Design review of the part built by this model. Coordinates are the model's own, in mm. A direction names the side the tool comes from. Coordinates: 2 decimals unless noted, no trailing zeros. Loops run counter-clockwise (first coordinate to the right, second up) from the corner with the lowest first, then second, coordinate; pieces in that order, holes last. Notation, with made-up numbers: (15.5, -8) -> (63.5, -8) arc R31 ccw to (63.5, 19) -> close; hole circle Ø6 at (70, 75.25). An arc over 180 degrees is marked (long way). Answer as a JSON object with one key per item and string values.
```python
from build123d import *

# Parameters (mm, degrees)
ESQUISSE2_R                  = 20.5
EXTRUSION1_DEPTH             = 4.8
ESQUISSE3_R                  = 6.25
EXTRUSION2_DEPTH             = 10
ENL_V_MAT_EXTRU_1_DEPTH      = 10
ESQUISSE5_R                  = 1.5
ENL_V_MAT_EXTRU_2_DEPTH      = 33.550576032
ESQUISSE6_R                  = 6.4
ENL_V_MAT_EXTRU_3_DEPTH      = 1.8
ESQUISSE7_R                  = 1
ENL_V_MAT_EXTRU_4_DEPTH      = 1
ENL_V_MAT_EXTRU_5_DEPTH      = 1.8
R_P_TITION_CIRCULAIRE1_COUNT = 6


with BuildPart() as part:
    # Esquisse2 → Extrusion1 (new body)
    with BuildSketch(Plane.XY):
        Circle(ESQUISSE2_R)
    extrude(amount=EXTRUSION1_DEPTH)

    # Esquisse3 → Extrusion2 (add)
    with BuildSketch(Plane.XY.offset(4.8)):
        with Locations((-3.25, 0)):
            Circle(ESQUISSE3_R)
    extrude(amount=EXTRUSION2_DEPTH)

    # Esquisse4 → Enl_v. mat.-Extru.1 (cut)
    with BuildSketch(Plane.XY.offset(14.8)):
        with BuildLine():
            ThreePointArc((0.388846154, 2.974693038), (-3, 0), (0.388846154, -2.974693038))
            ThreePointArc((0.388846154, -2.974693038), (-7.95, 0), (0.388846154, 2.974693038))
        make_face()
    extrude(amount=-ENL_V_MAT_EXTRU_1_DEPTH, mode=Mode.SUBTRACT)

    # Esquisse5 → Enl_v. mat.-Extru.2 (cut, through all)
    with BuildSketch(Plane.XY.offset(14.8)):
        Circle(ESQUISSE5_R)
    extrude(amount=-ENL_V_MAT_EXTRU_2_DEPTH, mode=Mode.SUBTRACT)

    # Esquisse6 → Enl_v. mat.-Extru.3 (cut)
    with BuildSketch(Plane(origin=(0, 0, 0), x_dir=(-1, 0, 0), z_dir=(0, 0, -1))):
        Circle(ESQUISSE6_R)
    extrude(amount=-ENL_V_MAT_EXTRU_3_DEPTH, mode=Mode.SUBTRACT)

    # Esquisse7 → Enl_v. mat.-Extru.4 (cut)
    with BuildSketch(Plane.XY.offset(4.8)):
        with Locations((0, 15)):
            Circle(ESQUISSE7_R)
    extrude(amount=-ENL_V_MAT_EXTRU_4_DEPTH, mode=Mode.SUBTRACT)

    # Esquisse8 → Enl_v. mat.-Extru.5 (cut)
    with BuildSketch(Plane(origin=(0, 0, 0), x_dir=(-1, 0, 0), z_dir=(0, 0, -1))):
        with BuildLine():
            Line((-3.190947925, 7.22688393), (-7.708190102, 15.05097689))
            ThreePointArc((-7.708190102, 15.05097689), (0, 16.91), (7.708190102, 15.05097689))
            Line((7.708190102, 15.05097689), (3.190947925, 7.22688393))
            ThreePointArc((3.190947925, 7.22688393), (0, 7.9), (-3.190947925, 7.22688393))
        make_face()
    enl_v_mat_extru_5 = extrude(amount=-ENL_V_MAT_EXTRU_5_DEPTH, mode=Mode.SUBTRACT)

    # R_p_tition circulaire1: Enl_v. mat.-Extru.5 ×6 about axis
    r_p_tition_circulaire1_axis = Axis((0, 0, 0), (0, 0, 1))
    for i in range(1, R_P_TITION_CIRCULAIRE1_COUNT):
        add(enl_v_mat_extru_5.rotate(r_p_tition_circulaire1_axis, i * 360 / R_P_TITION_CIRCULAIRE1_COUNT), mode=Mode.SUBTRACT)


solid = part.part
```
1) Add section C-C, the plane y = -18. Give the boundary of the cut face in (x, z), and give its area (3 significant figures).
Completed:
{"outline": "(-9.81, 0) -> (9.81, 0) -> (9.81, 4.8) -> (-9.81, 4.8) -> close", "area": "94.2 mm²"}
2) Add section B-B, the plane z = 10.25. Give the boundary of the cut face in (x, y).
Completed:
{"outline": "circle Ø12.5 at (-3.25, 0); hole circle Ø3 at (0, 0); hole (0.39, -2.97) arc R3 cw (long way) to (0.39, 2.97) arc R4.7 ccw (long way) to start"}
3) Add section A-A, the plane y = 0. Give the boundary of the cut face in (x, z), and give its area (3 significant figures).
Completed:
{"outline": "(-20.5, 0) -> (-6.4, 0) -> (-6.4, 1.8) -> (-1.5, 1.8) -> (-1.5, 14.8) -> (-3, 14.8) -> (-3, 4.8) -> (-7.95, 4.8) -> (-7.95, 14.8) -> (-9.5, 14.8) -> (-9.5, 4.8) -> (-20.5, 4.8) -> close; (1.5, 1.8) -> (6.4, 1.8) -> (6.4, 0) -> (20.5, 0) -> (20.5, 4.8) -> (3, 4.8) -> (3, 14.8) -> (1.5, 14.8) -> close", "area": "210 mm²"}
4) Clearance check with flat-ended pins moving along their axes: pin 1 Ø3 at (y, z) = (0, 9.5) entering from +X; pin 2 Ø0.5 at (x, z) = (13.5, 1.5) entering from +Y; pin 3 Ø3 at (x, y) = (0, 15) entering from -Z. State where each tip first meets the part, or that it passes through.
Completed:
{"pin 1": "x = 3", "pin 2": "y = 15.64", "pin 3": "z = 1.8"}
5) Wall thickness on probe 1 along Y at (x, z) = (0, 4.6); probe 2 along Y at (x, z) = (-2.5, 8); probe 3 along Y at (x, z) = (-0.5, 5.5): over which ranges is each line inside the solid? List them lowest first.
Completed:
{"probe 1": "-20.5 to -1.5, 1.5 to 14, 16 to 20.5", "probe 2": "-6.2 to -4.64, -1.66 to 1.66, 4.64 to 6.2", "probe 3": "-5.61 to -3.81, -2.96 to -1.41, 1.41 to 2.96, 3.81 to 5.61"}
6) For faces 1 (the flat face through (-2, 0, 14.8)), 2 (the cylindrical face through (14.7, 8.36, 0.89)), list the 3-axis set-ups (+Z, -Z, +X, -X, +Y, -Y) from which the entire face can be reached by the end or side of a thin tool; tool diameter is ignored.
Completed:
{"face 1": "+Z, +X, -X, +Y, -Y", "face 2": "-Z"}
7) The part is to be moulded in two halves that separate along Y. For faces 3 (the flat face through (-10, -6, 1.8)), 4 (the flat face through (4, 0, 4.8)), 5 (the cylindrical face through (-4.444, -20.013, 2.366)), say which applies: pulls with the +Y half, pulls with the -Y half, needs draft (parallel to the pull), parting line crosses it, or undercut.
Completed:
{"face 3": "undercut", "face 4": "needs draft", "face 5": "parting line crosses it"}
